from build123d import *

# Parameters (mm, degrees)
F0_R     = 41.7904194507
F1_DEPTH = 63.5
F3_DEPTH = 127.001


with BuildPart() as f1:
    # F0 (on Front) → F1 (new body, symmetric)
    with BuildSketch(Plane.XZ):
        with Locations((-9.8128121016, 15.3752699469)):
            Circle(F0_R)
    extrude(amount=F1_DEPTH, both=True)

    # F2 (on face) → F3 (cut, through all)
    with BuildSketch(Plane.XZ.offset(63.5)):
        Polygon((-25.5735145776, 20.9861662898), (-15.1132475585, 16.4628084749), (-22.1351497328, 25.825347257), align=None)
        Polygon((-30.5027123541, 14.048775658), (-25.5735145776, 20.9861662898), (-30.5027123541, 23.1177108519), align=None)
        Polygon((-30.5027123541, 23.1177108519), (-25.5735145776, 20.9861662898), (-22.1351497328, 25.825347257), (-26.2723503194, 31.341616208), (-30.5027123541, 29.3637841009), align=None)
        Polygon((-26.2723503194, 31.341616208), (-22.1351497328, 25.825347257), (-14.2079843208, 36.982100457), align=None)
        Polygon((-37.4430641532, 26.1189434677), (-30.5027123541, 23.1177108519), (-30.5027123541, 29.3637841009), align=None)
        Polygon((-30.5027123541, 29.3637841009), (-26.2723503194, 31.341616208), (-30.5027123541, 36.982100457), align=None)
    extrude(amount=-F3_DEPTH, mode=Mode.SUBTRACT)


solid = f1.part
Part model, mm, in its own coordinate system. Give positions to 0.01 mm unless a question says otherwise; leave off trailing zeros. Loops run counter-clockwise (first coordinate to the right, second up) from the corner with the lowest first, then second, coordinate; pieces in that order, holes last. Notation, with made-up numbers: (-15.5, -35.75) -> (-11.5, -35.75) arc R34 ccw to (-11.5, 3.25) -> close; hole circle Ø5 at (-31.75, 64). An arc over 180 degrees is marked (long way). Write each question's results on one line, items separated by ' | '. Start each with the question number.
Q1. Pin check, flat tips, straight feed: P1, Ø8, axis at x = -26.5, y = 8.5, coming from the +Z side; P2, Ø2, axis at x = 16.5, y = -27.5, coming from the +Z side; P3, Ø12, axis at y = 48, z = -17.5, coming from the -X side; P4, Ø4.5, axis at y = 3.5, z = 17, coming from the +X side. Stop position of each tip, or through.
Q2. Band-saw the part on C-C on z = 50. List the corners of the cut face in (x, y), plus the area to 3 significant figures.
Q3. Band-saw the part on A-A on x = -18.5. List the corners of the cut face in (y, z), plus the area to 3 significant figures.
Q4. Pull direction Z, two halves, no side cores. Call faces 1 (the face through (-28.07, -0.89, 17.47)), 2 (the face through (-10, -63.5, 16)), 3 (the face through (-40.614, -0.889, 43.619)): +Z half, -Z half, draft (parallel to the pull), parting line (faces both ways), or undercut.
Q5. Wall check: L1, parallel to Z at x = -17, y = -15.5; L2, parallel to Z at x = -21, y = 16; L3, parallel to Z at x = -32, y = -6. Give the ranges that are in metal, low to high.
Q6. Band-saw the part on D-D on x = 5. List the corners of the cut face in (y, z), plus the area to 3 significant figures.
Q7. Band-saw the part on B-B on y = 31.5. List the corners of the cut face in (x, z).
Results are:
1) P1: stops at z = 55.19 | P2: stops at z = 48.63 | P3: stops at x = -41.82 | P4: stops at x = 31.98
2) outline: (-33.21, -63.5) -> (13.59, -63.5) -> (13.59, 63.5) -> (-33.21, 63.5) -> close | area: 5,940 mm²
3) outline: (-63.5, -25.5) -> (63.5, -25.5) -> (63.5, 17.93) -> (-63.5, 17.93) -> close; (-63.5, 20.98) -> (63.5, 20.98) -> (63.5, 30.94) -> (-63.5, 30.94) -> close; (-63.5, 34.98) -> (63.5, 34.98) -> (63.5, 56.25) -> (-63.5, 56.25) -> close | area: 9,480 mm²
4) face 1: undercut | face 2: draft | face 3: parting line
5) L1: z = -25.79 to 17.28, 18.98 to 33.05, 35.68 to 56.54 | L2: z = -24.89 to 19.01, 24.31 to 27.42, 33.81 to 55.64 | L3: z = -20.04 to 23.77, 28.66 to 50.79
6) outline: (-63.5, -23.7) -> (63.5, -23.7) -> (63.5, 54.45) -> (-63.5, 54.45) -> close | area: 9,930 mm²
7) outline: circle Ø83.58 at (-9.81, 15.38); hole (-37.44, 26.12) -> (-30.5, 23.12) -> (-30.5, 14.05) -> (-25.57, 20.99) -> (-15.11, 16.46) -> (-22.14, 25.83) -> (-14.21, 36.98) -> (-26.27, 31.34) -> (-30.5, 36.98) -> (-30.5, 29.36) -> close
